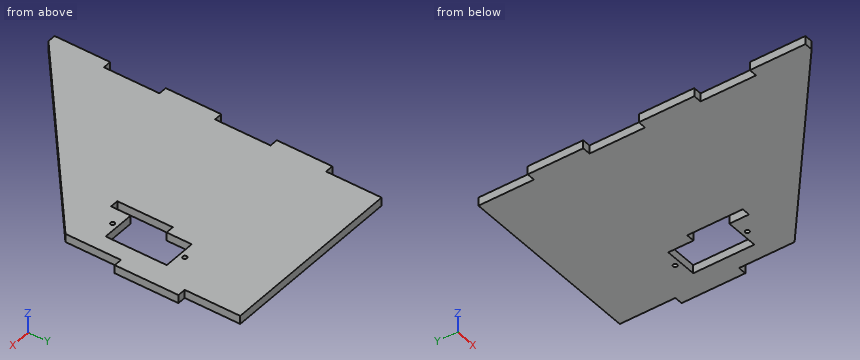
from build123d import *

# Parameters (mm, degrees)
SKETCH1_R           = 0.75
BOSS_EXTRUDE1_DEPTH = 3


with BuildPart() as part:
    # Sketch1 → Boss-Extrude1 (new body)
    with BuildSketch(Plane.XY):
        Polygon((-3, 60), (-3, 40), (0, 40), (0, 20), (-3, 20), (-3, 0), (0, 0), (68, 57.05877492), (68, 77.05877492), (71, 77.05877492), (71, 100), (68, 100), (68, 120), (23.5, 120), (0, 120), (0, 100), (-3, 100), (-3, 80), (0, 80), (0, 60), align=None)
        with Locations((56, 91.05877492)):
            Circle(SKETCH1_R, mode=Mode.SUBTRACT)
        with Locations(Location((56, 65.05877492, 0), (0, 0, 180))):
            Circle(SKETCH1_R, mode=Mode.SUBTRACT)
        Polygon((47, 80), (50, 80), (50, 89.05877492), (62, 89.05877492), (62, 67.05877492), (50, 67.05877492), (50, 60), (47, 60), align=None, mode=Mode.SUBTRACT)
    extrude(amount=BOSS_EXTRUDE1_DEPTH)


solid = part.part
Geometry: final body of the model. Coordinates: model frame, mm. Give positions to 0.01 mm unless a question says otherwise; leave off trailing zeros. Write each loop counter-clockwise with the first axis right and the second up, starting at its lowest first coordinate (ties: lowest second). Pieces come first, ordered by that corner, then holes. Notation, with made-up numbers: M -30,82 L 29,82 A22 cw 29,91 Z; hole C -28,-37.5 d11. An arc over 180 degrees is marked long. Answer in a Markdown table with one row per item. Add a question column.
(1) First-contact query: pin 1 (1.5 mm diameter, centred on y = 64.5, z = 2, fed in from -X); pin 2 (1.5 mm diameter, centred on x = -1.5, z = 1, fed in from +Y); pin 3 (0.9 mm diameter, centred on x = 69, z = 1.5, fed in from -Y). Flat tips, straight axial feed; report the tip coordinate or a pass-through.
(2) Section D-D on x = 11. Return loops of the section in (y, z).
(3) Section A-A on x = 53. Return loops of the section in (y, z).
(4) Section C-C on y = 109. Return loops of the section in (x, z), and give its area (3 significant figures).
(5) Section B-B on z = 2.3. State how many separate pieces and enclosed holes the cut face has, and give its area (3 significant figures).
(6) Ray query, line 1 (Y direction, x = 56, z = 1.8); line 2 (X direction, y = 74.5, z = 2.85); line 3 (X direction, y = 84, z = 1.05). Return the intervals inside material, ascending.
Result set:
| question | item | result |
|---|---|---|
| 1 | pin 1 | stops at x = 0 |
| 1 | pin 2 | stops at y = 100 |
| 1 | pin 3 | stops at y = 77.06 |
| 2 | outline | M 9.23,0 L 120,0 L 120,3 L 9.23,3 Z |
| 3 | outline | M 44.47,0 L 67.06,0 L 67.06,3 L 44.47,3 Z; M 89.06,0 L 120,0 L 120,3 L 89.06,3 Z |
| 4 | outline | M 0,0 L 68,0 L 68,3 L 0,3 Z |
| 4 | area | 204 mm^2 |
| 5 | separate pieces | 1 |
| 5 | enclosed holes | 3 |
| 5 | area | 6,140 mm^2 |
| 6 | line 1 | y = 46.99 to 64.31, 65.81 to 67.06, 89.06 to 90.31, 91.81 to 120 |
| 6 | line 2 | x = 0 to 47, 62 to 68 |
| 6 | line 3 | x = -3 to 50, 62 to 71 |
